For this review, take the finished solid that the model builds, in its own axes (mm). A direction names the side the tool comes from. Coordinates: 2 decimals unless noted, no trailing zeros. Loops run counter-clockwise (first coordinate to the right, second up) from the corner with the lowest first, then second, coordinate; pieces in that order, holes last. Notation, with made-up numbers: M 0,20.5 L 29,20.5 A34 ccw 29,59.5 Z; hole C 80.5,-27 d1. An arc over 180 degrees is marked long. Use one line per item in the form item = value.
```python
from build123d import *

# Parameters (mm, degrees)
PAD005_DEPTH    = 11.25
SKETCH036_W     = 20.5
SKETCH036_H     = 6.6332701871
POCKET002_DEPTH = 24.5032991847
POCKET003_DEPTH = 1


with BuildPart() as part:
    # Sketch035 → Pad005 (new body, symmetric)
    with BuildSketch(Plane.YZ):
        with BuildLine():
            ThreePointArc((13.3821850753, -37.5234542499), (18.3608599681, -33.5666154319), (20.5067387818, -27.5800486999))
            ThreePointArc((24.3536477534, -28.4698782284), (22.9530190653, -25.7646841778), (20.5067387818, -27.5800486999))
            ThreePointArc((13.4426775015, -37.713318887), (20.0290903971, -34.4265472751), (24.3536477534, -28.4698782284))
            ThreePointArc((13.3821850753, -37.5234542499), (13.3252924513, -37.6461497146), (13.4426775015, -37.713318887))
        make_face()
    extrude(amount=PAD005_DEPTH, both=True)

    # Sketch036 → Pocket002 (cut, through all)
    with BuildSketch(Plane.XZ):
        with Locations((0, -28.8966837934)):
            Rectangle(SKETCH036_W, SKETCH036_H)
        with BuildLine():
            ThreePointArc((-12.5299423012, -36.4092487677), (0, -37.463318887), (12.5299423012, -36.4092487677))
            Line((12.5299423012, -40.220734), (12.5299423012, -36.4092487677))
            Line((-12.5299423012, -40.220734), (12.5299423012, -40.220734))
            Line((-12.5299423012, -36.4092487677), (-12.5299423012, -40.220734))
        make_face()
    extrude(amount=-POCKET002_DEPTH, mode=Mode.SUBTRACT)

    # Sketch037 → Pocket003 (cut, symmetric)
    with BuildSketch(Plane.YZ):
        with BuildLine():
            Line((22.16829374, -32.213318887), (21.46829374, -32.213318887))
            Line((21.46829374, -32.213318887), (21.46829374, -33.0380523289))
            ThreePointArc((21.46829374, -33.0380523289), (21.8254978862, -32.6318001925), (22.16829374, -32.213318887))
        make_face()
    extrude(amount=POCKET003_DEPTH, both=True, mode=Mode.SUBTRACT)


solid = part.part
```
1. Consider section C-C on y = 20.25. Write out the cut boundary in (x, z).
Computed values:
outline = M -11.25,-34.24 L 11.25,-34.24 L 11.25,-29.35 L 10.25,-29.35 L 10.25,-32.21 L -10.25,-32.21 L -10.25,-29.35 L -11.25,-29.35 Z
2. For pin 1 Ø3 at (x, z) = (8, -35) entering from -Y; pin 2 Ø1 at (x, z) = (-1, -32) entering from -Y; pin 3 Ø5 at (x, z) = (5, -31.5) entering from +Y; pin 4 Ø5 at (x, z) = (-5, -29) entering from +Y, all flat-tipped, find the tip position at first contact; note any pin that passes through.
Computed values:
pin_1 = 15.31
pin_2 = 19.04
pin_3 = 22.17
pin_4 = through
3. Consider section D-D on x = 2.5. Write out the cut boundary in (y, z), plus the area to 3 significant figures.
Computed values:
outline = M 13.62,-37.42 L 14.54,-37.42 A15.48 ccw 22.17,-32.21 L 19.2,-32.21 A11.61 cw Z
area = 11.2 mm2
4. Draft analysis for pull direction X (two halves, no side actions). For faces 1 (the face through (-0.158, 14.02, -37.463)), 2 (the face through (-11.25, 21, -30)), 3 (the face through (-10.743, 23, -25.776)), 4 (the face through (0, 21, -32.213)), state which applies: +X half, -X half, draft (parallel to the pull), parting line (faces both ways), or undercut.
Computed values:
face_1 = parting line
face_2 = -X half
face_3 = draft
face_4 = undercut
5. Consider section A-A on z = -30.25. Write out the cut boundary in (x, y), plus the area to 3 significant figures.
Computed values:
outline = M -11.25,20.01 L -10.25,20.01 L -10.25,23.49 L -11.25,23.49 Z; M 10.25,20.01 L 11.25,20.01 L 11.25,23.49 L 10.25,23.49 Z
area = 6.96 mm2
6. Tool access review of faces 5 (the face through (0.158, 17.461, -34.672)), 6 (the face through (-10.25, 22, -29)), 7 (the face through (0, 21.468, -32.6)): name each direction out of +Z, -Z, +X, -X, +Y, -Y from which nothing blocks a thin tool from reaching the whole face with its end or side.
Computed values:
face_5 = +Z, +X, -X, -Y
face_6 = +Z, +Y, -Y
face_7 = +Z, -Z, +Y
7. Consider section B-B on y = 23.75. Write out the cut boundary in (x, z), plus the area to 3 significant figures.
Computed values:
outline = M -11.25,-29.77 L -10.25,-29.77 L -10.25,-26.15 L -11.25,-26.15 Z; M 10.25,-29.77 L 11.25,-29.77 L 11.25,-26.15 L 10.25,-26.15 Z
area = 7.24 mm2
8. Wall thickness on line 1 along X through (y, z) = (21.75, -26.5); line 2 along Z through (x, y) = (-0.5, 14); line 3 along Y through (x, z) = (3.25, -35.25): over which ranges is each line inside the solid? List them lowest first. Write a range as from..to.
Computed values:
line_1 = -11.25..-10.25, 10.25..11.25
line_2 = -37.46..-37.25
line_3 = 16.89..18.97
